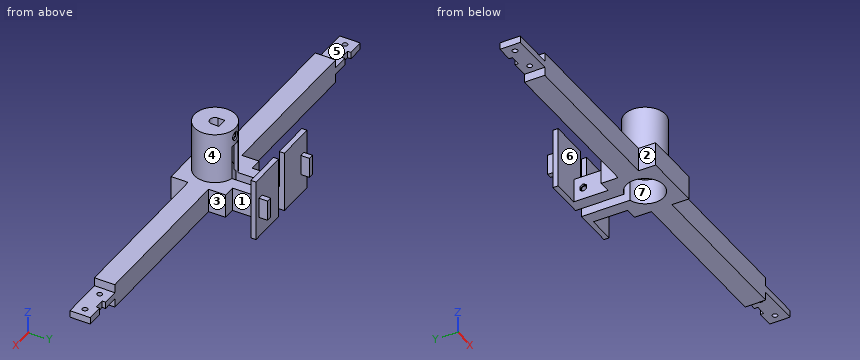
from build123d import *

# Parameters (mm, degrees)
BOSS_EXTRUDE1_DEPTH = 14
SKETCH2_R           = 12
BOSS_EXTRUDE2_DEPTH = 30
CUT_EXTRUDE2_DEPTH  = 34
BOSS_EXTRUDE3_START = 19
BOSS_EXTRUDE3_DEPTH = 19
CUT_EXTRUDE3_DEPTH  = 149.789280528
SKETCH10_R          = 1.5
CUT_EXTRUDE5_DEPTH  = 148.87241122
CUT_EXTRUDE6_DEPTH  = 1.5
CUT_EXTRUDE7_REACH  = 160.077
SKETCH12_R          = 1.5
SKETCH13_R          = 2.5
CUT_EXTRUDE8_DEPTH  = 1
CUT_EXTRUDE9_DEPTH  = 1
SKETCH15_W          = 25
SKETCH15_H          = 5
CUT_EXTRUDE11_DEPTH = 148.452534766
CUT_EXTRUDE12_START = -5.5
SKETCH17_R          = 2.5
CUT_EXTRUDE12_DEPTH = 143.055074494
SKETCH18_W          = 23
SKETCH18_H          = 36
BOSS_EXTRUDE7_DEPTH = 3
SKETCH19_W          = 3.1
SKETCH19_H          = 12
BOSS_EXTRUDE8_DEPTH = 5
SKETCH21_R          = 1.5
SKETCH21_W          = 6
SKETCH21_H          = 2
CUT_EXTRUDE13_DEPTH = 149.550496489


with BuildPart() as part:
    # Sketch1 → Boss-Extrude1 (new body)
    with BuildSketch(Plane.XY):
        Polygon((10, 16), (17, 16), (17, 6), (137.5, 6), (137.5, -6), (17, -6), (17, -16), (-17, -16), (-17, -6), (-137.5, -6), (-137.5, 6), (-17, 6), (-17, 16), (-10, 16), (-10, 36), (10, 36), align=None)
    extrude(amount=BOSS_EXTRUDE1_DEPTH)

    # Sketch2 → Boss-Extrude2 (add)
    with BuildSketch(Plane.XY.offset(14)):
        Circle(SKETCH2_R)
    extrude(amount=BOSS_EXTRUDE2_DEPTH)

    # Sketch5 → Cut-Extrude2 (cut)
    with BuildSketch(Plane(origin=(0, 0, 0), x_dir=(-1, 0, 0), z_dir=(0, 0, -1))):
        with BuildLine():
            Line((-3, 36), (-3, 10.583005244))
            ThreePointArc((-3, 10.583005244), (0, -11), (3, 10.583005244))
            Line((3, 10.583005244), (3, 36))
            Line((3, 36), (-3, 36))
        make_face()
    extrude(amount=-CUT_EXTRUDE2_DEPTH, mode=Mode.SUBTRACT)

    # Sketch7 → Boss-Extrude3 (add)
    with BuildSketch(Plane(origin=(0, 0, 34), x_dir=(-1, 0, 0), z_dir=(0, 0, -1)).offset(BOSS_EXTRUDE3_START)):
        with BuildLine():
            Line((-3, 10.583005244), (-3, 9.539392014))
            ThreePointArc((-3, 9.539392014), (0, -10), (3, 9.539392014))
            Line((3, 9.539392014), (3, 10.583005244))
            ThreePointArc((3, 10.583005244), (0, -11), (-3, 10.583005244))
        make_face()
    extrude(amount=-BOSS_EXTRUDE3_DEPTH)

    # Sketch6 → Cut-Extrude3 (cut, through all)
    with BuildSketch(Plane.XY.offset(44)):
        with BuildLine():
            Line((-3, 0), (-3, 4))
            Line((-3, 4), (3, 4))
            Line((3, 4), (3, 0))
            ThreePointArc((3, 0), (0, -3), (-3, 0))
        make_face()
    extrude(amount=-CUT_EXTRUDE3_DEPTH, mode=Mode.SUBTRACT)

    # Sketch10 → Cut-Extrude5 (cut, through all)
    with BuildSketch(Plane(origin=(0, 4, 0), x_dir=(-1, 0, 0), z_dir=(0, -1, 0))):
        with Locations(Location((0, -39, 0), (0, 0, 90))):
            Circle(SKETCH10_R)
    extrude(amount=-CUT_EXTRUDE5_DEPTH, mode=Mode.SUBTRACT)

    # Sketch11 → Cut-Extrude6 (cut)
    with BuildSketch(Plane.XZ.offset(-4)):
        Polygon((2, 37.845299462), (2, 40.154700538), (0, 41.309401077), (-2, 40.154700538), (-2, 37.845299462), (0, 36.690598923), align=None)
    extrude(amount=-CUT_EXTRUDE6_DEPTH, mode=Mode.SUBTRACT)

    # Cut-Extrude7: up to this face of the body (flat: up to its plane)
    cut_extrude7_end = Plane(part.part.faces().sort_by_distance((-10, 26, 7))[0])
    # Sketch12 → Cut-Extrude7 (cut, up to the picked face)
    with BuildSketch(Plane(origin=(10, 0, 0), x_dir=(0, 0, -1), z_dir=(1, 0, 0)), mode=Mode.PRIVATE) as cut_extrude7_sk1:
        with Locations(Location((-7, 30.5, 0), (0, 0, 90))):
            Circle(SKETCH12_R)
    cut_extrude7_tool1 = split(extrude(cut_extrude7_sk1.sketch, amount=-CUT_EXTRUDE7_REACH, mode=Mode.PRIVATE), bisect_by=cut_extrude7_end, keep=Keep.BOTH, mode=Mode.PRIVATE)
    add(cut_extrude7_tool1.solids().sort_by(Axis((10, 30.5, 7), (-1, 0, 0)))[0], mode=Mode.SUBTRACT)

    # Sketch13 → Cut-Extrude8 (cut)
    with BuildSketch(Plane(origin=(10, 0, 0), x_dir=(0, 0, -1), z_dir=(1, 0, 0))):
        with Locations(Location((-7, 30.5, 0), (0, 0, 90))):
            Circle(SKETCH13_R)
    extrude(amount=-CUT_EXTRUDE8_DEPTH, mode=Mode.SUBTRACT)

    # Sketch14 → Cut-Extrude9 (cut)
    with BuildSketch(Plane.ZY.offset(10)):
        Polygon((4.690598923, 30.5), (5.845299462, 28.5), (8.154700538, 28.5), (9.309401077, 30.5), (8.154700538, 32.5), (5.845299462, 32.5), align=None)
    extrude(amount=-CUT_EXTRUDE9_DEPTH, mode=Mode.SUBTRACT)

    # Sketch15 → Cut-Extrude11 (cut, through all)
    with BuildSketch(Plane(origin=(0, 6, 0), x_dir=(1, 0, 0), z_dir=(0, 1, 0))):
        with Locations((-125, -11.5)):
            Rectangle(SKETCH15_W, SKETCH15_H)
        with Locations((-125, -2.5)):
            Rectangle(SKETCH15_W, SKETCH15_H)
    cut_extrude11 = extrude(amount=-CUT_EXTRUDE11_DEPTH, mode=Mode.SUBTRACT)

    # Mirror2: Cut-Extrude11 across plane
    add(cut_extrude11.mirror(Plane(origin=(0, 0, 0), x_dir=(0, 0, 1), z_dir=(1, 0, 0))), mode=Mode.SUBTRACT)

    # Sketch17 → Cut-Extrude12 (cut, through all)
    with BuildSketch(Plane.XZ.offset(-5.5).offset(CUT_EXTRUDE12_START)):
        with Locations(Location((0, 39, 0), (0, 0, 270))):
            Circle(SKETCH17_R)
    extrude(amount=-CUT_EXTRUDE12_DEPTH, mode=Mode.SUBTRACT)

    # Sketch18 → Boss-Extrude7 (add)
    with BuildSketch(Plane(origin=(0, 36, 0), x_dir=(1, 0, 0), z_dir=(0, 1, 0))):
        with Locations((-14.5, -18)):
            Rectangle(SKETCH18_W, SKETCH18_H)
        with Locations((14.5, -18)):
            Rectangle(SKETCH18_W, SKETCH18_H)
    extrude(amount=BOSS_EXTRUDE7_DEPTH)

    # Sketch19 → Boss-Extrude8 (add)
    with BuildSketch(Plane(origin=(0, 39, 0), x_dir=(1, 0, 0), z_dir=(0, 1, 0))):
        with Locations((-21.4, -18)):
            Rectangle(SKETCH19_W, SKETCH19_H)
        with Locations((21.4, -18)):
            Rectangle(SKETCH19_W, SKETCH19_H)
    extrude(amount=BOSS_EXTRUDE8_DEPTH)

    # Sketch21 → Cut-Extrude13 (cut, through all)
    with BuildSketch(Plane.XY.offset(9)):
        with Locations((-132.5, 0)):
            Circle(SKETCH21_R)
        with Locations((-117.5, 0)):
            Circle(SKETCH21_R)
        with Locations((-125, 5)):
            Rectangle(SKETCH21_W, SKETCH21_H)
    cut_extrude13 = extrude(amount=-CUT_EXTRUDE13_DEPTH, mode=Mode.SUBTRACT)

    # Mirror3: Cut-Extrude13 across plane
    add(cut_extrude13.mirror(Plane(origin=(0, 0, 0), x_dir=(0, 0, 1), z_dir=(1, 0, 0))), mode=Mode.SUBTRACT)


solid = part.part
Check sheet for the modelled part. Datum: model origin and axes. Units: mm. Face numbers are marked on the shaded views. A direction names the side the tool comes from. Round coordinates to 2 decimals unless told otherwise and drop trailing zeros. Loops run counter-clockwise (first coordinate to the right, second up) from the corner with the lowest first, then second, coordinate; pieces in that order, holes last. Notation, with made-up numbers: (54.25, 46.5) - (69.25, 46.5) arc R10 cw to (69.25, 57.5) - close; hole circle Ø9 at (30.25, 57). An arc over 180 degrees is marked (long way). Answer as CSV lines item,"result". Start each with the question number.
Item 1: Release check for a two-part mould opening along Y. For the marked faces 1 and 2 record: +Y half, -Y half, draft (parallel to the pull), parting line (faces both ways), or undercut.
Item 2: Section check B-B (x = 57.5). Record the boundary of the cut face in (y, z).
Item 3: Depth check by flat-ended pin: P1, Ø12, axis at y = -9, z = 18.5, coming from the -X side; P2, Ø7, axis at y = 28.5, z = 10, coming from the +X side; P3, Ø2, axis at y = 24, z = 11, coming from the -X side. Enter the tip coordinate at first touch or a pass-through.
Item 4: Set-up check for the marked faces 3, 4, 5, 6 and 7: record each of +Z, -Z, +X, -X, +Y, -Y from which the full face is reachable in a straight line by a thin tool's end or side.
Item 5: Section check A-A (z = 21.5). Record the boundary of the cut face in (x, y).
Item 6: Scan lines: line 1 (Z direction, x = -5.8, y = 30.5); line 2 (Y direction, x = 4, z = 30.5); line 3 (Y direction, x = -121, z = 8). Record each from-to range of solid material in increasing order. Write a range as [from, to].
Report:
1,face 1,"undercut"
1,face 2,"draft"
2,outline,"(-6, 0) - (6, 0) - (6, 14) - (-6, 14) - close"
3,P1,"stops at x = -112.5"
3,P2,"stops at x = 10"
3,P3,"stops at x = -10"
4,face 3,"+Z, -Z, +X"
4,face 4,"+Z"
4,face 5,"+Z, -X, +Y, -Y"
4,face 6,"+Z, -X"
4,face 7,"-Z"
5,outline,"(-26, 36) - (-3, 36) - (-3, 39) - (-19.85, 39) - (-19.85, 44) - (-22.95, 44) - (-22.95, 39) - (-26, 39) - close; (-3, 9.54) - (-3, 11.62) arc R12 ccw (long way) to (3, 11.62) - (3, 9.54) arc R10 cw (long way) to start; (3, 36) - (26, 36) - (26, 39) - (22.95, 39) - (22.95, 44) - (19.85, 44) - (19.85, 39) - (3, 39) - close"
6,line 1,"z = [0, 5.5], [8.5, 14]"
6,line 2,"y = [-11.31, -9.17], [9.17, 11.31], [36, 39]"
6,line 3,"y = [-6, 6]"
